from build123d import *

# Parameters (mm, degrees)
F0_R     = 1.6
F1_DEPTH = 10


with BuildPart() as f1:
    # F0 (on Top) → F1 (new body)
    with BuildSketch(Plane.XY):
        with BuildLine():
            Line((20, 36), (0, 36))
            Line((0, 36), (-20, 36))
            ThreePointArc((-20, 36), (-22.828427, 34.828427), (-24, 32))
            Line((-24, 32), (-24, 0))
            Line((-24, 0), (-24, -32))
            ThreePointArc((-24, -32), (-22.828427, -34.828427), (-20, -36))
            Line((-20, -36), (0, -36))
            Line((0, -36), (20, -36))
            ThreePointArc((20, -36), (22.828427, -34.828427), (24, -32))
            Line((24, -32), (24, 0))
            Line((24, 0), (24, 32))
            ThreePointArc((24, 32), (22.828427, 34.828427), (20, 36))
        make_face()
        with Locations((-19, -30)):
            Circle(F0_R, mode=Mode.SUBTRACT)
        with Locations((19, -30)):
            Circle(F0_R, mode=Mode.SUBTRACT)
        with Locations((-19, 30)):
            Circle(F0_R, mode=Mode.SUBTRACT)
        with Locations((19, 30)):
            Circle(F0_R, mode=Mode.SUBTRACT)
    extrude(amount=F1_DEPTH)


solid = f1.part
Read the model definition and answer for the solid it produces. Units are mm, in the model's axes. Give positions to 0.01 mm unless a question says otherwise; leave off trailing zeros. Loops run counter-clockwise (first coordinate to the right, second up) from the corner with the lowest first, then second, coordinate; pieces in that order, holes last. Notation, with made-up numbers: M 34,31 L 80,31 A28 cw 80,65 Z; hole C 75,-19 d3. An arc over 180 degrees is marked long. Write each question's results on one line, items separated by ' | '.
1. Straight lines are drawn through the part: line 1 (Y direction, x = -19, z = 6); line 2 (X direction, y = 31, z = 8.5); line 3 (Y direction, x = -22, z = 4.25). For each, find the intervals that lie inside material, in ascending order. Write a range as [from, to].
Values:
line 1: y = [-36, -31.6], [-28.4, 28.4], [31.6, 36] | line 2: x = [-24, -20.25], [-17.75, 17.75], [20.25, 24] | line 3: y = [-35.46, 35.46]
2. Section A-A on x = -19 is taken. Give the vertices of the cut face in (y, z).
Values:
outline: M -36,0 L -31.6,0 L -31.6,10 L -36,10 Z; M -28.4,0 L 28.4,0 L 28.4,10 L -28.4,10 Z; M 31.6,0 L 36,0 L 36,10 L 31.6,10 Z
3. Section B-B on y = -30 is taken. Give the vertices of the cut face in (x, z).
Values:
outline: M -24,0 L -20.6,0 L -20.6,10 L -24,10 Z; M -17.4,0 L 17.4,0 L 17.4,10 L -17.4,10 Z; M 20.6,0 L 24,0 L 24,10 L 20.6,10 Z
